from build123d import *

# Parameters (mm, degrees)
CROQUIS2_W              = 37.219606625
CROQUIS2_H              = 25.289645753
SALIENTE_EXTRUIR1_DEPTH = 5
CROQUIS3_W              = 12.822792139
CROQUIS3_H              = 10.241869911
SALIENTE_EXTRUIR2_DEPTH = 60
CROQUIS4_W              = 2
CROQUIS4_H              = 6.778219121
CORTAR_EXTRUIR1_DEPTH   = 60
CORTAR_EXTRUIR2_REACH   = 263.618
CROQUIS5_R              = 1.85
CROQUIS6_R              = 1.85
CORTAR_EXTRUIR3_DEPTH   = 74.340748192


with BuildPart() as part:
    # Croquis2 → Saliente-Extruir1 (new body)
    with BuildSketch(Plane.XY):
        with Locations((10.975865795, -240.275746154)):
            Rectangle(CROQUIS2_W, CROQUIS2_H)
    extrude(amount=SALIENTE_EXTRUIR1_DEPTH)

    # Croquis3 → Saliente-Extruir2 (add)
    with BuildSketch(Plane.XY.offset(5)):
        with Locations((-1.222541449, -241.35158101)):
            Rectangle(CROQUIS3_W, CROQUIS3_H)
    extrude(amount=SALIENTE_EXTRUIR2_DEPTH)

    # Croquis4 → Cortar-Extruir1 (cut)
    with BuildSketch(Plane.ZY.offset(7.633937518)):
        with Locations((37, -239.446035793)):
            Rectangle(CROQUIS4_W, CROQUIS4_H)
    extrude(amount=-CORTAR_EXTRUIR1_DEPTH, mode=Mode.SUBTRACT)

    # Croquis5 → Cortar-Extruir2 (cut, up to next)
    with BuildSketch(Plane.XY.offset(5), mode=Mode.PRIVATE) as cortar_extruir2_sk1:
        with Locations((-2.795177489, -249.862416258)):
            Circle(CROQUIS5_R)
    cortar_extruir2_tool1 = extrude(cortar_extruir2_sk1.sketch, amount=-CORTAR_EXTRUIR2_REACH, mode=Mode.PRIVATE) & part.part
    # Croquis5 → Cortar-Extruir2 (cut, up to next)
    with BuildSketch(Plane.XY.offset(5), mode=Mode.PRIVATE) as cortar_extruir2_sk2:
        with Locations((22.369152578, -245.40207204)):
            Circle(CROQUIS5_R)
    cortar_extruir2_tool2 = extrude(cortar_extruir2_sk2.sketch, amount=-CORTAR_EXTRUIR2_REACH, mode=Mode.PRIVATE) & part.part
    add(cortar_extruir2_tool1.solids().sort_by_distance((-2.795177, -249.862416, 5))[0], mode=Mode.SUBTRACT)
    add(cortar_extruir2_tool2.solids().sort_by_distance((22.369153, -245.402072, 5))[0], mode=Mode.SUBTRACT)

    # Croquis6 → Cortar-Extruir3 (cut, through all)
    with BuildSketch(Plane(origin=(0, -236.230646054, 0), x_dir=(1, 0, 0), z_dir=(0, 1, 0))):
        with Locations(Location((1.905498405, -58.778240746, 0), (0, 0, 270))):
            Circle(CROQUIS6_R)
        with Locations(Location((-4.523066348, -58.778240746, 0), (0, 0, 270))):
            Circle(CROQUIS6_R)
    extrude(amount=-CORTAR_EXTRUIR3_DEPTH, mode=Mode.SUBTRACT)


solid = part.part
Model file for the job. Use its own axes, mm. A direction names the side the tool comes from. Give positions to 0.01 mm unless a question says otherwise; leave off trailing zeros. Write each loop counter-clockwise with the first axis right and the second up, starting at its lowest first coordinate (ties: lowest second). Pieces come first, ordered by that corner, then holes. Notation, with made-up numbers: M 53.5,33.5 L 81.5,33.5 A25 ccw 81.5,56.5 Z; hole C 76,8 d3. An arc over 180 degrees is marked long. One line per item, written item: value. Start each with the question number.
Q1. Probe probe 1 along Z at (x, y) = (-4.5, -239.25); probe 2 along Z at (x, y) = (5, -233.75); probe 3 along X at (y, z) = (-245.5, 45.5). List the from-to ranges inside material, lowest first. Write a range as [from, to].
Q2. Saw through at C-C, the plane z = 37. Write the cut outline in (x, y), plus the area to 3 significant figures.
Q3. Saw through at B-B, the plane y = -248.75. Write the cut outline in (x, z).
Q4. Two-plate mould, pull along X, no slides. Class faces 6 (the flat face through (29.586, -240, 2)), 7 (the flat face through (11, -252.921, 2)), 8 (the cylindrical face through (-3.04, -248.03, 2.54)): +X half, -X half, draft (parallel to the pull), parting line (faces both ways), or undercut.
Q5. Saw through at A-A, the plane y = -239.5. Write the cut outline in (x, z), plus the area to 3 significant figures.
Q6. Drop flat-ended pins along their axis: pin 1 Ø12 at (y, z) = (-232, 17) entering from +X; pin 2 Ø4 at (x, z) = (-1.5, 15) entering from +Y; pin 3 Ø5 at (x, y) = (-2.8, -249.86) entering from +Z; pin 4 Ø3 at (x, y) = (22.37, -245.4) entering from +Z. Give the stop position or say it passes through.
Q7. 3-axis set-ups, long thin cutter, end or side, ignore diameter. For faces 1 (the flat face through (-1, -236.231, 20)), 2 (the flat face through (11, -227.631, 2)), 3 (the flat face through (-1, -246.473, 35)), 4 (the flat face through (5.189, -241, 35)), 5 (the flat face through (-1, -240, 38)): which of +Z, -Z, +X, -X, +Y, -Y reach the whole face in a straight line?
Q8. Saw through at D-D, the plane x = 12.5. Write the cut outline in (y, z).
Output values:
1. probe 1: z = [0, 36], [38, 56.93], [60.63, 65]
1. probe 2: z = [0, 5]
1. probe 3: x = [-7.63, 5.19]
2. outline: M -7.63,-246.47 L 5.19,-246.47 L 5.19,-242.84 L -7.63,-242.84 Z
2. area: 46.6 mm²
3. outline: M -7.63,0 L -4.27,0 L -4.27,5 L -7.63,5 Z; M -1.32,0 L 29.59,0 L 29.59,5 L -1.32,5 Z
4. face 6: +X half
4. face 7: draft
4. face 8: undercut
5. outline: M -7.63,0 L 29.59,0 L 29.59,5 L 5.19,5 L 5.19,36 L -7.63,36 Z; M -7.63,38 L 5.19,38 L 5.19,65 L -7.63,65 Z; hole C -4.52,58.78 d3.7; hole C 1.91,58.78 d3.7
5. area: 908 mm²
6. pin 1: stops at x = 5.19
6. pin 2: stops at y = -236.23
6. pin 3: stops at z = 5
6. pin 4: passes through
7. face 1: +Z, +X, -X, +Y
7. face 2: +Z, -Z, +X, -X, +Y
7. face 3: +Z, +X, -X, -Y
7. face 4: +Z, +X, +Y, -Y
7. face 5: +X, -X, +Y
8. outline: M -252.92,0 L -227.63,0 L -227.63,5 L -252.92,5 Z
